```python
from build123d import *

# Parameters (mm, degrees)
F0_W     = 76.2
F0_H     = 457.2
F1_DEPTH = 19.05
F3_DEPTH = 19.051
F4_SIZE  = 19.04999


# Not quite as in the source:
# - a fillet or chamfer is up to 0.001 mm smaller than in the source, because OpenCascade refuses the exact size


with BuildPart() as f1:
    # F0 (on Front) → F1 (new body)
    with BuildSketch(Plane.XZ):
        with Locations((38.1, 228.6)):
            Rectangle(F0_W, F0_H)
    extrude(amount=F1_DEPTH)

    # F2 (on face) → F3 (cut, through all)
    with BuildSketch(Plane.XZ.offset(19.05)):
        Polygon((0, 355.6), (28.575, 457.2), (0, 457.2), align=None)
        Polygon((76.2, 457.2), (47.625, 457.2), (76.2, 355.6), align=None)
    extrude(amount=-F3_DEPTH, mode=Mode.SUBTRACT)

    # F4 (size 19.05 in the source; OpenCascade refuses exactly that, so slightly less here)
    f4_edges = [f1.edges().sort_by_distance(p)[0] for p in [
        (38.1, -19.05, 457.2),
    ]]
    chamfer(f4_edges, length=F4_SIZE)


solid = f1.part
```
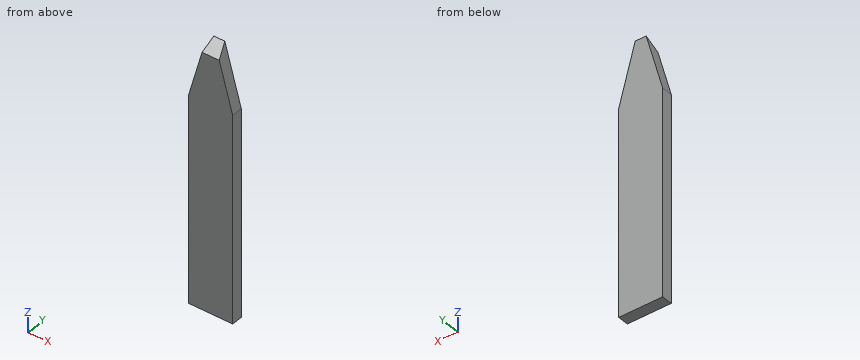
Input: part model. Units: mm. Frame: model coordinates. Round coordinates to 2 decimals unless told otherwise and drop trailing zeros. Loops run counter-clockwise (first coordinate to the right, second up) from the corner with the lowest first, then second, coordinate; pieces in that order, holes last. Notation, with made-up numbers: (-20.75, 36) -> (-5.75, 36) arc R19 ccw to (-5.75, 71) -> close; hole circle Ø3 at (-37.5, 40). An arc over 180 degrees is marked (long way). Use one line per item in the form item = value. Start each with the question number.
Item 1: Section query A-A on x = 64.5. Return the cut outline in (y, z), then the cut area to 3 significant figures.
Item 2: Contact query for flat-ended pins moving along their axis: pin 1 Ø4 at (x, y) = (33, -6.5) entering from +Z; pin 2 Ø10 at (x, y) = (55, -16) entering from +Z; pin 3 Ø6 at (x, y) = (39, -11.5) entering from +Z. Output: stop coordinate, or through.
Item 3: Section query C-C on z = 372.5. Return the cut outline in (x, y), then the cut area to 3 significant figures.
Item 4: Material intervals for L1, parallel to Z at x = 42, y = -2; L2, parallel to X at y = -3.25, z = 407; L3, parallel to Z at x = 29, y = -8, sorted ascending. Write a range as from..to.
Item 5: Section query B-B on y = -4.5. Return the cut outline in (x, z), then the cut area to 3 significant figures.
Ans:
q1.outline = (-19.05, 0) -> (0, 0) -> (0, 397.2) -> (-19.05, 397.2) -> close
q1.area = 7,570 mm^2
q2.pin_1 = 452.7
q2.pin_2 = 444.46
q2.pin_3 = 448.7
q3.outline = (4.75, -19.05) -> (71.45, -19.05) -> (71.45, 0) -> (4.75, 0) -> close
q3.area = 1,270 mm^2
q4.L1 = 0..455.2
q4.L2 = 14.46..61.74
q4.L3 = 0..449.2
q5.outline = (0, 0) -> (76.2, 0) -> (76.2, 355.6) -> (48.89, 452.7) -> (27.31, 452.7) -> (0, 355.6) -> close
q5.area = 31,800 mm^2
